from build123d import *

# Parameters (mm, degrees)
HEADDISPLAYBRACKET_THICKNESS_DEPTH = 17.78
SKETCH3_R                          = 2.54
CUT_EXTRUDE1_DEPTH                 = 17.78


with BuildPart() as part:
    # HeadDisplayBraceOutline → HeadDisplayBracket_Thickness (new body)
    with BuildSketch(Plane.XY):
        with BuildLine():
            Line((137.16, -6013.450000001), (-603.25, -6013.450000001))
            Line((-603.25, -6013.450000001), (-603.25, -5867.400000001))
            Line((-603.25, -5867.400000001), (-155.878238141, -5867.400000001))
            ThreePointArc((-155.878238141, -5867.400000001), (-141.328560309, -5864.951302064), (-128.38193157, -5857.875))
            ThreePointArc((-128.38193157, -5857.875), (-115.435302831, -5850.798697937), (-100.885625, -5848.35))
            Line((-100.885625, -5848.35), (-50.085625, -5848.35))
            ThreePointArc((-50.085625, -5848.35), (-35.535947169, -5850.798697937), (-22.58931843, -5857.875))
            ThreePointArc((-22.58931843, -5857.875), (-9.642689691, -5864.951302063), (4.906988141, -5867.400000001))
            Line((4.906988141, -5867.400000001), (137.16, -5867.400000001))
            Line((137.16, -5867.400000001), (137.16, -6013.450000001))
        make_face()
    extrude(amount=-HEADDISPLAYBRACKET_THICKNESS_DEPTH)

    # Sketch3 → Cut-Extrude1 (cut)
    with BuildSketch(Plane.XY):
        with Locations((-333.454375, -5994.4)):
            Circle(SKETCH3_R)
        with Locations((-132.635625, -5994.4)):
            Circle(SKETCH3_R)
        with Locations((-132.635625, -5894.07)):
            Circle(SKETCH3_R)
        with Locations((-333.454375, -5894.07)):
            Circle(SKETCH3_R)
        with BuildLine():
            Line((-104.060625, -5892.8), (-104.060625, -5969))
            ThreePointArc((-104.060625, -5969), (-103.13068903, -5971.24506403), (-100.885625, -5972.175))
            Line((-100.885625, -5972.175), (-50.085625, -5972.175))
            ThreePointArc((-50.085625, -5972.175), (-47.84056097, -5971.24506403), (-46.910625, -5969))
            Line((-46.910625, -5969), (-46.910625, -5892.8))
            Line((-46.910625, -5892.8), (-50.085625, -5889.625))
            Line((-50.085625, -5889.625), (-100.885625, -5889.625))
            ThreePointArc((-100.885625, -5889.625), (-103.13068903, -5890.55493597), (-104.060625, -5892.8))
        make_face()
    extrude(amount=-CUT_EXTRUDE1_DEPTH, mode=Mode.SUBTRACT)


solid = part.part
Model file for the job. Use its own axes, mm. A direction names the side the tool comes from. Give positions to 0.01 mm unless a question says otherwise; leave off trailing zeros. Loops run counter-clockwise (first coordinate to the right, second up) from the corner with the lowest first, then second, coordinate; pieces in that order, holes last.
Item 1: Which spindle directions (+Z, -Z, +X, -X, +Y, -Y) get a long thin tool onto all of the face, cutting with end or side? Do faces 1 (the face through (-383, -5867.4, -9)), 2 (the face through (-75, -5889.625, -9)), 3 (the face through (-76, -5848.35, -9)). Say none if no direction does.
Check values:
face 1: +Z, -Z, -X, +Y
face 2: +Z, -Z
face 3: +Z, -Z, +X, -X, +Y
Item 2: Slice it at A-A (x = -70). Write the cut outline in (y, z) (3 decimals).
Check values:
outline: (-6013.45, -17.78) - (-5972.175, -17.78) - (-5972.175, 0) - (-6013.45, 0) - close; (-5889.625, -17.78) - (-5848.35, -17.78) - (-5848.35, 0) - (-5889.625, 0) - close
Item 3: Slice it at B-B (y = -5962). Write the cut outline in (x, z).
Check values:
outline: (-603.25, -17.78) - (-104.06, -17.78) - (-104.06, 0) - (-603.25, 0) - close; (-46.91, -17.78) - (137.16, -17.78) - (137.16, 0) - (-46.91, 0) - close
Item 4: Drop flat-ended pins along their axis: P1, Ø4, axis at x = -132.64, y = -5894.07, coming from the +Z side (3 decimals); P2, Ø5.5, axis at x = -385, z = -13, coming from the +Y side. Give the stop position or say it passes through.
Check values:
P1: passes through
P2: stops at y = -5867.4
Item 5: Drill centre lines: line 1 along X through (y, z) = (-5894.07, -4.5); line 2 along X through (y, z) = (-5994.5, -10.75); line 3 along X through (y, z) = (-5938, -4.5). Where is each one in solid material? Low to high.
Check values:
line 1: x = -603.25 to -335.99, -330.91 to -135.18, -130.1 to -104.06, -46.91 to 137.16
line 2: x = -603.25 to -335.99, -330.92 to -135.17, -130.1 to 137.16
line 3: x = -603.25 to -104.06, -46.91 to 137.16
Item 6: Slice it at C-C (z = -6.25). Write the cut outline in (x, y) (3 decimals), plus the area to 3 significant figures.
Check values:
outline: (-603.25, -6013.45) - (137.16, -6013.45) - (137.16, -5867.4) - (4.907, -5867.4) arc R44.45 cw to (-22.589, -5857.875) arc R44.45 ccw to (-50.086, -5848.35) - (-100.886, -5848.35) arc R44.45 ccw to (-128.382, -5857.875) arc R44.45 cw to (-155.878, -5867.4) - (-603.25, -5867.4) - close; hole circle Ø5.08 at (-333.454, -5994.4); hole circle Ø5.08 at (-333.454, -5894.07); hole circle Ø5.08 at (-132.636, -5994.4); hole circle Ø5.08 at (-132.636, -5894.07); hole (-104.061, -5969) arc R3.175 ccw to (-100.886, -5972.175) - (-50.086, -5972.175) arc R3.175 ccw to (-46.911, -5969) - (-46.911, -5892.8) - (-50.086, -5889.625) - (-100.886, -5889.625) arc R3.175 ccw to (-104.061, -5892.8) - close
area: 105,000 mm2
Item 7: Slice it at D-D (x = 57). Write the cut outline in (y, z), plus the area to 3 significant figures.
Check values:
outline: (-6013.45, -17.78) - (-5867.4, -17.78) - (-5867.4, 0) - (-6013.45, 0) - close
area: 2,600 mm2
Item 8: Mould opens along X. For faces 4 (the face through (70, -5867.4, -9)), 5 (the face through (-46.911, -5931, -9)), 6 (the face through (-603.25, -5941, -9)) say: +X half, -X half, draft (parallel to the pull), parting line (faces both ways), or undercut.
Check values:
face 4: draft
face 5: undercut
face 6: -X half
